Study the drawing (mm; zero at the part's minimum x, y, z) and answer. A direction names the side the tool comes from. Coordinates: 2 decimals unless noted, no trailing zeros. Order: outer loops, then holes, each group sorted by start corner. A loop starts at its lowest first (then second) coordinate and runs counter-clockwise, first axis right, second up. Notation, with made-up numbers: (46.5, -32) - (59.5, -32) arc R16 ccw to (59.5, -9) - close; hole circle Ø10 at (44.25, -29). An arc over 180 degrees is marked (long way). Write item = value, one per line.
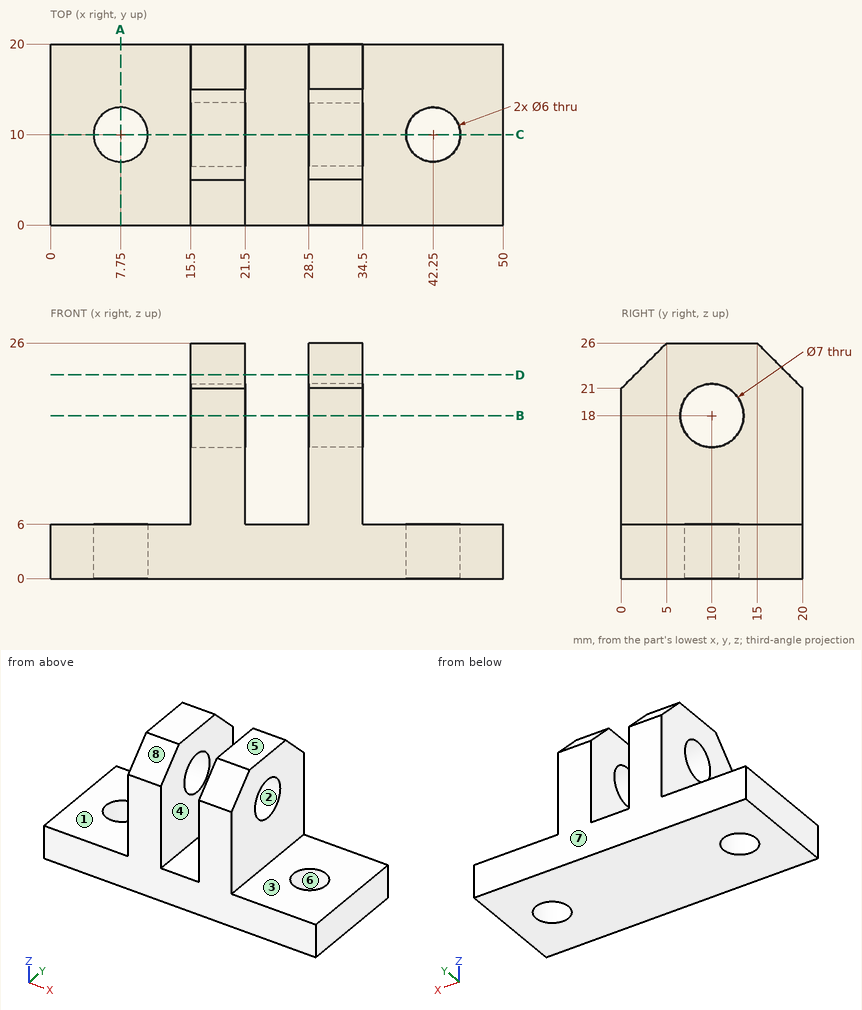
1) Flat-ended cylindrical pins translate along their axes: pin 1 Ø7 at (x, y) = (7.75, 10) entering from +Z; pin 2 Ø10 at (y, z) = (12.5, 3.5) entering from -X; pin 3 Ø10 at (y, z) = (6.5, 16.5) entering from -X; pin 4 Ø11 at (y, z) = (10, 18) entering from +X. Find the tip coordinate at first contact, or state that the pin passes through.
Returned:
pin_1 = 6
pin_2 = 0
pin_3 = 15.5
pin_4 = 34.5
2) The part is cut by section D-D (z = 22.5). Determine the outline of the cut face in (x, y).
Returned:
outline = (15.5, 1.5) - (21.5, 1.5) - (21.5, 18.5) - (15.5, 18.5) - close; (28.5, 1.5) - (34.5, 1.5) - (34.5, 18.5) - (28.5, 18.5) - close
3) The part is cut by section B-B (z = 18). Determine the outline of the cut face in (x, y).
Returned:
outline = (15.5, 0) - (21.5, 0) - (21.5, 6.5) - (15.5, 6.5) - close; (15.5, 13.5) - (21.5, 13.5) - (21.5, 20) - (15.5, 20) - close; (28.5, 0) - (34.5, 0) - (34.5, 6.5) - (28.5, 6.5) - close; (28.5, 13.5) - (34.5, 13.5) - (34.5, 20) - (28.5, 20) - close
4) The part is cut by section A-A (x = 7.75). Determine the outline of the cut face in (y, z).
Returned:
outline = (0, 0) - (7, 0) - (7, 6) - (0, 6) - close; (13, 0) - (20, 0) - (20, 6) - (13, 6) - close
5) Determine the mould class of the marked faces 5, 6, 7 and 8 for opening direction Y: pulls with the +Y half, pulls with the -Y half, needs draft (parallel to the pull), parting line crosses it, or undercut.
Returned:
face_5 = needs draft
face_6 = undercut
face_7 = pulls with the +Y half
face_8 = pulls with the -Y half
6) The part is cut by section C-C (y = 10). Determine the outline of the cut face in (x, z), and give its area (3 significant figures).
Returned:
outline = (0, 0) - (4.75, 0) - (4.75, 6) - (0, 6) - close; (10.75, 0) - (39.25, 0) - (39.25, 6) - (34.5, 6) - (34.5, 14.5) - (28.5, 14.5) - (28.5, 6) - (21.5, 6) - (21.5, 14.5) - (15.5, 14.5) - (15.5, 6) - (10.75, 6) - close; (15.5, 21.5) - (21.5, 21.5) - (21.5, 26) - (15.5, 26) - close; (28.5, 21.5) - (34.5, 21.5) - (34.5, 26) - (28.5, 26) - close; (45.25, 0) - (50, 0) - (50, 6) - (45.25, 6) - close
area = 384 mm^2
7) Straight lines are drawn through the part: line 1 along Z through (x, y) = (16.8, 10); line 2 along Y through (x, z) = (7.75, 2); line 3 along X through (y, z) = (5.75, 23.25). For each, find the intervals that lie inside material, in ascending order. Write a range as from..to.
Returned:
line_1 = 0..14.5, 21.5..26
line_2 = 0..7, 13..20
line_3 = 15.5..21.5, 28.5..34.5
8) For the marked faces 1, 2, 3 and 4, determine the directions among +Z, -Z, +X, -X, +Y, -Y from which every point of the face is accessible in a straight line to the end or side of a thin tool.
Returned:
face_1 = +Z, -X, +Y, -Y
face_2 = +X, -X
face_3 = +Z, +X, +Y, -Y
face_4 = +Z, +Y, -Y
